The listing builds one solid part. Answer for the finished solid, in the listing's coordinates (mm). A direction names the side the tool comes from. Give positions to 0.01 mm unless a question says otherwise; leave off trailing zeros. Write each loop counter-clockwise with the first axis right and the second up, starting at its lowest first coordinate (ties: lowest second). Pieces come first, ordered by that corner, then holes.
```python
from build123d import *

# Parameters (mm, degrees)
SKETCH1_R               = 11.5
SKETCH1_R_2             = 5
BOSS_EXTRUDE1_DEPTH     = 20
CUT_EXTRUDE1_DEPTH      = 7
CUT_EXTRUDE2_DEPTH      = 26.777897509
CUT_EXTRUDE2_DEPTH_BACK = 26.777897509
SKETCH3_W               = 8
SKETCH3_H               = 16
BOSS_EXTRUDE2_START     = -4
SKETCH4_R               = 20
SKETCH4_R_2             = 11.5
BOSS_EXTRUDE2_DEPTH     = 4


with BuildPart() as part:
    # Sketch1 → Boss-Extrude1 (new body)
    with BuildSketch(Plane.XY):
        Circle(SKETCH1_R)
        Circle(SKETCH1_R_2, mode=Mode.SUBTRACT)
    extrude(amount=BOSS_EXTRUDE1_DEPTH)

    # Sketch2 → Cut-Extrude1 (cut)
    with BuildSketch(Plane.XY.offset(20)):
        Polygon((8, 0), (4, 6.92820323), (-4, 6.92820323), (-8, 0), (-4, -6.92820323), (4, -6.92820323), align=None)
    extrude(amount=-CUT_EXTRUDE1_DEPTH, mode=Mode.SUBTRACT)

    # Sketch3 → Cut-Extrude2 (cut, two sides: drawn at the far end of the back side and taken through both)
    with BuildSketch(Plane(origin=(0, 0, 0), x_dir=(0, 0, -1), z_dir=(1, 0, 0)).offset(-CUT_EXTRUDE2_DEPTH_BACK)):
        with Locations((-4, 0)):
            Rectangle(SKETCH3_W, SKETCH3_H)
    extrude(amount=CUT_EXTRUDE2_DEPTH + CUT_EXTRUDE2_DEPTH_BACK, mode=Mode.SUBTRACT)

    # Sketch4 → Boss-Extrude2 (add)
    with BuildSketch(Plane.XY.offset(20).offset(BOSS_EXTRUDE2_START)):
        Circle(SKETCH4_R)
        with Locations(Location((0, 0, 0), (0, 0, 135.920790152))):
            Circle(SKETCH4_R_2, mode=Mode.SUBTRACT)
    extrude(amount=BOSS_EXTRUDE2_DEPTH)


solid = part.part
```
Item 1: A cutting plane is placed at A-A, the plane z = 19. Give the vertices of the cut face in (x, y), plus the area to 3 significant figures.
Conclusion:
outline: circle Ø40 at (0, 0); hole (-8, 0) - (-4, -6.93) - (4, -6.93) - (8, 0) - (4, 6.93) - (-4, 6.93) - close
area: 1,090 mm2
Item 2: Determine the mould class of faces 1 (the face through (5, -2, 8)), 2 (the face through (10.97, 3.45, 9.67)), 3 (the face through (5.972, -3.513, 16.549)) for opening direction X: pulls with the +X half, pulls with the -X half, needs draft (parallel to the pull), parting line crosses it, or undercut.
Conclusion:
face 1: needs draft
face 2: parting line crosses it
face 3: undercut
Item 3: Each of these flat-tipped pins is pushed along its axis until it touches: P1, Ø8, axis at x = -11, y = -3, coming from the -Z side; P2, Ø12, axis at x = 8.5, y = -9, coming from the -Z side; P3, Ø9, axis at x = 1.5, z = 4.5, coming from the -Y side; P4, Ø7.5, axis at x = -2, z = 17, coming from the +Y side. Where does it stop, or does it pass through?
Conclusion:
P1: stops at z = 8
P2: stops at z = 0
P3: stops at y = -11.5
P4: stops at y = 20
Item 4: A cutting plane is placed at B-B, the plane x = 0. Give the vertices of the cut face in (y, z).
Conclusion:
outline: (-20, 16) - (-11.5, 16) - (-11.5, 0) - (-8, 0) - (-8, 8) - (-5, 8) - (-5, 13) - (-6.93, 13) - (-6.93, 20) - (-20, 20) - close; (5, 8) - (8, 8) - (8, 0) - (11.5, 0) - (11.5, 16) - (20, 16) - (20, 20) - (6.93, 20) - (6.93, 13) - (5, 13) - close
Item 5: A cutting plane is placed at C-C, the plane y = 1.5. Give the vertices of the cut face in (x, z), plus the area to 3 significant figures.
Conclusion:
outline: (-19.94, 16) - (-11.4, 16) - (-11.4, 8) - (-4.77, 8) - (-4.77, 13) - (-7.13, 13) - (-7.13, 20) - (-19.94, 20) - close; (4.77, 8) - (11.4, 8) - (11.4, 16) - (19.94, 16) - (19.94, 20) - (7.13, 20) - (7.13, 13) - (4.77, 13) - close
area: 194 mm2
Item 6: Which of the six approach directions +Z, -Z, +X, -X, +Y, -Y give full straight-line access (tool end or side, diameter ignored) to faces 4 (the face through (0, -9, 0)), 5 (the face through (0, 6.928, 17)), 6 (the face through (0, 8, 4)), 7 (the face through (-4.336, -19.524, 17.972)), 8 (the face through (9, -9, 16))?
Conclusion:
face 4: -Z, +X, -X, +Y, -Y
face 5: +Z
face 6: -Z, +X, -X
face 7: +Z, -Z
face 8: -Z
Item 7: Consider probe 1 along Y at (x, z) = (0, 11.8); probe 2 along Z at (x, y) = (6, -10.5). Determine where each line is inside the solid, lowest interval first.
Conclusion:
probe 1: y = -11.5 to -5, 5 to 11.5
probe 2: z = 16 to 20
Item 8: A cutting plane is placed at D-D, the plane z = 15.25. Give the vertices of the cut face in (x, y), plus the area to 3 significant figures.
Conclusion:
outline: circle Ø23 at (0, 0); hole (-8, 0) - (-4, -6.93) - (4, -6.93) - (8, 0) - (4, 6.93) - (-4, 6.93) - close
area: 249 mm2
